The listing builds one solid part. Answer for the finished solid, in the listing's coordinates (mm). Face numbers are marked on the shaded views. A direction names the side the tool comes from. Round coordinates to 2 decimals unless told otherwise and drop trailing zeros. Loops run counter-clockwise (first coordinate to the right, second up) from the corner with the lowest first, then second, coordinate; pieces in that order, holes last. Notation, with made-up numbers: M 22.25,69.5 L 72.25,69.5 A15 ccw 72.25,85.5 Z; hole C 44,27.25 d10. An arc over 180 degrees is marked long. Put each result on its own line as item: value. Start each with the question number.
(1) Section D-D, the plane x = -33 is taken. Determine the outline of the cut face in (y, z).
(2) Section A-A, the plane x = 16 is taken. Determine the outline of the cut face in (y, z), then the cut area to 3 significant figures.
(3) Section B-B, the plane z = 10.25 is taken. Determine the outline of the cut face in (x, y).
(4) Determine the mould class of the marked faces 1, 2 and 3 for opening direction Z: released by +Z, released by -Z, zero draft, split by the parting line, or undercut.
(5) Flat-ended cylindrical pins translate along their axes: P1, Ø0.5, axis at y = 0, z = 13, coming from the -X side; P2, Ø8, axis at x = -16.5, z = 8, coming from the +Y side; P3, Ø0.5, axis at x = -3, z = 13, coming from the +Y side; P4, Ø4, axis at x = -9.5, y = -3.5, coming from the +Z side. Find the tip coordinate at first contact, or state that the pin passes through.
(6) Which of the six approach directions +Z, -Z, +X, -X, +Y, -Y give full straight-line access (tool end or side, diameter ignored) to the marked faces 4 and 5?
(7) Straight lines are drawn through the part: line 1 (Z direction, x = 18.5, y = -7); line 2 (Y direction, x = 11, z = 4.75); line 3 (X direction, y = 10, z = 7.25). For each, find the intervals that lie inside material, in ascending order.
(8) Section C-C, the plane y = 17 is taken. Determine the outline of the cut face in (x, z).
```python
from build123d import *

# Parameters (mm, degrees)
SKETCH1_W           = 43
SKETCH1_H           = 21.6
BOSS_EXTRUDE1_DEPTH = 14
SKETCH2_W           = 27.35
SKETCH2_H           = 18.3
CUT_EXTRUDE1_DEPTH  = 2
SKETCH3_W           = 7.85
SKETCH3_H           = 17.94
CUT_EXTRUDE2_DEPTH  = 8
REVOLVE2_ANGLE      = 90
SKETCH5_W           = 92.23581066
SKETCH5_H           = 73.43389541
SKETCH5_W_2         = 43
SKETCH5_H_2         = 21.6
CUT_EXTRUDE3_DEPTH  = 23
SKETCH6_R           = 2.105
SKETCH6_R_2         = 0.81
BOSS_EXTRUDE2_DEPTH = 1.3
SKETCH7_R           = 2.105
SKETCH7_R_2         = 0.81
BOSS_EXTRUDE3_DEPTH = 1.3
SKETCH8_R           = 0.81
BOSS_EXTRUDE4_DEPTH = 20
SKETCH9_R           = 0.815150105
BOSS_EXTRUDE5_DEPTH = 26
FILLET1_R           = 0.5


with BuildPart() as part:
    # Sketch1 → Boss-Extrude1 (new body)
    with BuildSketch(Plane.XY):
        Rectangle(SKETCH1_W, SKETCH1_H)
    extrude(amount=BOSS_EXTRUDE1_DEPTH)

    # Sketch2 → Cut-Extrude1 (cut)
    with BuildSketch(Plane.XY.offset(14)):
        with Locations((-6.175, 0)):
            Rectangle(SKETCH2_W, SKETCH2_H)
    extrude(amount=-CUT_EXTRUDE1_DEPTH, mode=Mode.SUBTRACT)

    # Sketch3 → Cut-Extrude2 (cut)
    with BuildSketch(Plane(origin=(21.5, 0, 0), x_dir=(0, 0, -1), z_dir=(1, 0, 0))):
        with Locations((-7.925, 0)):
            Rectangle(SKETCH3_W, SKETCH3_H)
    extrude(amount=-CUT_EXTRUDE2_DEPTH, mode=Mode.SUBTRACT)

    # Sketch4 → Revolve2 (revolve)
    with BuildSketch(Plane(origin=(0, -9.15, 0), x_dir=(1, 0, 0), z_dir=(0, 1, 0))):
        with BuildLine():
            Line((-32.583466089, -10.1469511), (-32.583466089, -12.265551486))
            add(Edge.make_bspline(
                [(-32.583466089, -12.265551486), (-32.562502483, -12.265551486), (-32.520421916, -12.266006033), (-32.4432028, -12.268051491), (-32.333162226, -12.273488053), (-32.204458453, -12.283626191), (-32.058326628, -12.301036433), (-31.883418572, -12.328702131), (-31.686720457, -12.369661846), (-31.491837838, -12.419079982), (-31.298991654, -12.47598715), (-31.074449095, -12.55061405), (-30.819301893, -12.645650497), (-30.534581384, -12.762541391), (-30.220087155, -12.900547222), (-29.829076239, -13.077316326), (-29.358834293, -13.28780702), (-28.785809577, -13.519520804), (-28.090562481, -13.719040931), (-27.293796046, -13.805648084), (-26.419142059, -13.693362453), (-25.49136496, -13.369953032), (-24.502198634, -12.908600866), (-23.392162802, -12.415282136), (-22.124309457, -12.154525407), (-20.858041285, -12.40646563), (-19.751906697, -12.893751072), (-18.769192416, -13.353235169), (-17.846551628, -13.682182536), (-16.973609278, -13.804616553), (-16.009305612, -13.711847073), (-15.005547104, -13.37431948), (-14.04749388, -12.909101), (-13.049418653, -12.482723934), (-12.133440252, -12.262513677), (-11.3353156, -12.242983824), (-10.409800826, -12.421010141), (-9.400945989, -12.826034613), (-8.434871057, -13.30301482), (-7.417140082, -13.675236005), (-6.457099181, -13.803910561), (-5.606473079, -13.72128943), (-4.682813704, -13.427765218), (-3.69904901, -12.975867192), (-2.756532087, -12.543833591), (-1.795314434, -12.273179903), (-0.966070624, -12.243102783), (-0.315946216, -12.343671298), (0.265672195, -12.515998278), (0.783591987, -12.717624267), (1.405691454, -12.993439328), (2.136134729, -13.329294572), (2.847403799, -13.604786677), (3.551966265, -13.750324658), (4.099646321, -13.773217429), (4.475706664, -13.751363619), (4.917058627, -13.680358163), (5.404652636, -13.54933903), (5.879870794, -13.370834982), (6.304903895, -13.187020764), (6.697517429, -13.011274996), (6.938033599, -12.90064266), (7.234652875, -12.773222965), (7.35452597, -12.722686103), (7.41653391, -12.697417231)],
                knots=[0.083339346, 0.083339346, 0.083339346, 0.083339346, 0.083339346, 0.085336612, 0.087333879, 0.089331145, 0.091328411, 0.095322944, 0.099317476, 0.103312008, 0.107306541, 0.111301073, 0.115295606, 0.122119207, 0.128942808, 0.13576641, 0.142590011, 0.156237213, 0.169884416, 0.18488454, 0.199884664, 0.219547445, 0.239210226, 0.26281996, 0.286429695, 0.316430056, 0.339777495, 0.363124933, 0.382799659, 0.402474385, 0.417474496, 0.432474606, 0.459256287, 0.486037969, 0.502278436, 0.518518903, 0.53373395, 0.548948997, 0.576756025, 0.604563053, 0.61956323, 0.634563408, 0.65321264, 0.671861872, 0.696234785, 0.720607698, 0.735607914, 0.750608131, 0.761649817, 0.772691503, 0.783733188, 0.794774874, 0.815713505, 0.836652137, 0.844152286, 0.851652435, 0.859152585, 0.866652734, 0.879411498, 0.892170261, 0.898549642, 0.904929024, 0.911308406, 0.917687787, 0.917687787, 0.917687787, 0.917687787, 0.917687787], degree=4))
            Line((7.41653391, -12.697417231), (7.41653391, -10.1469511))
            Line((7.41653391, -10.1469511), (-32.583466089, -10.1469511))
        make_face()
    revolve(axis=Axis((7.5, -9.15, 12), (0, 0, -1)), revolution_arc=REVOLVE2_ANGLE)

    # Sketch5 → Cut-Extrude3 (cut)
    with BuildSketch(Plane.XY):
        with Locations((3.214998373, 5.833103881)):
            Rectangle(SKETCH5_W, SKETCH5_H)
        Rectangle(SKETCH5_W_2, SKETCH5_H_2, mode=Mode.SUBTRACT)
    extrude(amount=CUT_EXTRUDE3_DEPTH, mode=Mode.SUBTRACT)

    # Sketch6 → Boss-Extrude2 (add)
    with BuildSketch(Plane.ZY.offset(21.5)):
        with Locations(Location((4.5, -5.8, 0), (0, 0, 180))):
            Circle(SKETCH6_R)
        with Locations((4.5, -5.8)):
            Circle(SKETCH6_R_2, mode=Mode.SUBTRACT)
    extrude(amount=BOSS_EXTRUDE2_DEPTH)

    # Sketch7 → Boss-Extrude3 (add)
    with BuildSketch(Plane(origin=(0, 10.8, -10.8), x_dir=(1, 0, 0), z_dir=(0, -1, 0))):
        with Locations(Location((-17, 15.3, 0), (0, 0, 270))):
            Circle(SKETCH7_R)
        with Locations(Location((-17, 15.3, 0), (0, 0, 270))):
            Circle(SKETCH7_R_2, mode=Mode.SUBTRACT)
    extrude(amount=-BOSS_EXTRUDE3_DEPTH)

    # Sketch8 → Boss-Extrude4 (add)
    with BuildSketch(Plane.ZY.offset(21.5)):
        with Locations((4.5, -5.8)):
            Circle(SKETCH8_R)
    extrude(amount=BOSS_EXTRUDE4_DEPTH)

    # Sketch9 → Boss-Extrude5 (add)
    with BuildSketch(Plane(origin=(0, 10.8, 0), x_dir=(1, 0, 0), z_dir=(0, 1, 0))):
        with Locations(Location((-17, -4.5, 0), (0, 0, 90))):
            Circle(SKETCH9_R)
    extrude(amount=BOSS_EXTRUDE5_DEPTH)

    # Fillet1
    fillet1_edges = [part.edges().sort_by_distance(p)[0] for p in [
        (-21.5, -10.8, 7),
        (0, -10.8, 14),
        (21.5, -10.8, 7),
        (0, 10.8, 0),
        (-21.5, 0, 0),
        (0, -10.8, 0),
        (21.5, 0, 0),
        (7.5, -9.15, 13),
        (7.5, 9.15, 13.179370152),
        (-19.85, 9.15, 13.656100765),
        (-19.85, -9.15, 13.428261731),
        (-21.5, 0, 14),
        (-21.5, 10.8, 7),
        (0, 10.8, 14),
        (21.5, 10.8, 7),
        (21.5, 0, 14),
    ]]
    fillet(fillet1_edges, radius=FILLET1_R)


solid = part.part
```
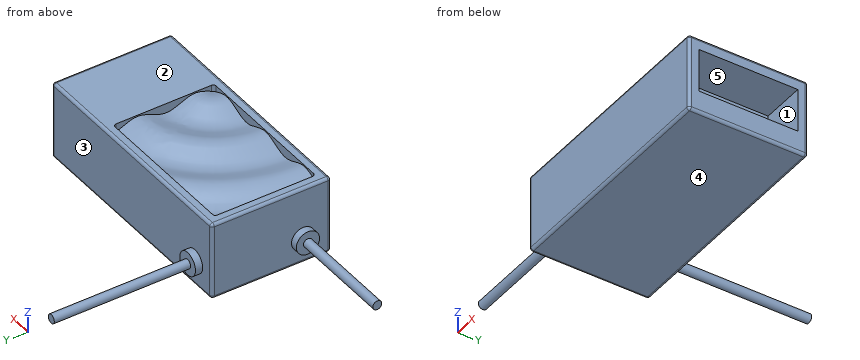
Recorded:
1. outline: C -5.8,4.5 d1.62
2. outline: M -10.8,0.5 A0.5 ccw -10.3,0 L 10.3,0 A0.5 ccw 10.8,0.5 L 10.8,13.5 A0.5 ccw 10.3,14 L -10.3,14 A0.5 ccw -10.8,13.5 Z; hole M -8.97,4 L 8.97,4 L 8.97,11.85 L -8.97,11.85 Z
2. area: 161 mm²
3. outline: M -21.5,-10.3 A0.5 ccw -21,-10.8 L 21,-10.8 A0.5 ccw 21.5,-10.3 L 21.5,-8.97 L 13.5,-8.97 L 13.5,8.97 L 21.5,8.97 L 21.5,10.3 A0.5 ccw 21,10.8 L -21,10.8 A0.5 ccw -21.5,10.3 Z
4. face 1: undercut
4. face 2: released by +Z
4. face 3: zero draft
5. P1: stops at x = -21.5
5. P2: stops at y = 36.8
5. P3: stops at y = 10.8
5. P4: stops at z = 13.28
6. face 4: -Z, +X, -X, +Y, -Y
6. face 5: +X
7. line 1: z = 0 to 4, 11.85 to 14
7. line 2: y = -10.8 to 10.8
7. line 3: x = -21.5 to 21.5
8. outline: C -17,4.5 d1.63
